Solid Edge part; units mm, degrees
sketch "Sketch1" plane through (0, 0, 0) normal (0, 0, 1) x (1, 0, 0)
  line L0 (4, -30) -> (4, 30)
  arc A0 (4, 30) -> (-1, 33.873) centre (0, 30) ccw
  line L1 (-2.5, 69.8417) -> (-1, 33.873)
  arc A1 (-2.5, 69.8417) -> (0.8311, 73.8267) centre (1.3567, 70.0026) cw
  arc A2 (0.6137, 75) -> (0.8311, 73.8267) centre (0.66, 74.4018) cw
  arc A3 (-4, 70.0149) -> (0.6137, 75) centre (1, 70.0149) cw
  line L2 (-4, 30) -> (-4, 70.0149)
  line L3 (-4, 30) -> (-4, -30)
  arc A4 (-4, -30) -> (4, -30) centre (0, -30) ccw
  dimension "D1" = 4
  dimension "D2" = 2.5
  dimension "D3" = 2.5
extrude "Ajout_matière_1" add sketch "Sketch1" along normal blind 1
sketch "Sketch2" plane through (0, 0, 0) normal (0, 0, 1) x (1, 0, 0)
  circle A0 centre (0, -30) radius 2
extrude "Cutout1" cut sketch "Sketch2" along normal up to next
properties material "Acier S235"
Check sheet for the modelled part. Datum: model origin and axes. Units: mm. A direction names the side the tool comes from. Give positions to 0.01 mm unless a question says otherwise; leave off trailing zeros. Write each loop counter-clockwise with the first axis right and the second up, starting at its lowest first coordinate (ties: lowest second). Pieces come first, ordered by that corner, then holes. Notation, with made-up numbers: M 55.5,39 L 72.5,39 A8 ccw 72.5,44 Z; hole C -32,12.25 d9. An arc over 180 degrees is marked long. Use one line per item in the form item = value.
(1) Material ranges on line 1 along X through (y, z) = (-30, 0.55); line 2 along Y through (x, z) = (0, 0.6); line 3 along Y through (x, z) = (-0.25, 0.85), recorded low to high.
Answer block:
line_1 = -4 to -2, 2 to 4
line_2 = -34 to -32, -28 to 34, 73.62 to 74.91
line_3 = -33.99 to -31.98, -28.02 to 33.99, 73.51 to 74.86
(2) Section check A-A on z = 0.45. Record the boundary of the cut face in (x, y).
Answer block:
outline = M -4,-30 A4 ccw 4,-30 L 4,30 A4 ccw -1,33.87 L -2.5,69.84 A3.86 cw 0.83,73.83 A0.6 ccw 0.61,75 A5 ccw -4,70.01 Z; hole C 0,-30 d4
(3) Tool access check on faces 1 (the cylindrical face through (-2.705, 73.373, 0.493)), 2 (the cylindrical face through (-1.63, 72.45, 0.49)). Record the directions out of +Z, -Z, +X, -X, +Y, -Y that give a thin tool (end or side, any length) a straight path to the whole face; none if there is none.
Answer block:
face_1 = +Z, -Z, -X, +Y
face_2 = +Z, -Z, +X
(4) Section check B-B on y = 52. Record the boundary of the cut face in (x, z), plus the area to 3 significant figures.
Answer block:
outline = M -4,0 L -1.76,0 L -1.76,1 L -4,1 Z
area = 2.24 mm2
(5) Draft check along Y on faces 3 (the cylindrical face through (0.1, -34, 0.5)), 4 (the flat face through (-1, 9, 0)), 5 (the cylindrical face through (-0.434, -28.048, 0.493)). Enter one of: pulls with the +Y half, pulls with the -Y half, needs draft (parallel to the pull), parting line crosses it, or undercut.
Answer block:
face_3 = pulls with the -Y half
face_4 = needs draft
face_5 = undercut
